Design review of the part shown in the three views and the two pictorial views. Dimensions are in mm from the part's minimum x, y and z. A direction names the side the tool comes from. Round coordinates to 2 decimals unless told otherwise and drop trailing zeros. Loops run counter-clockwise (first coordinate to the right, second up) from the corner with the lowest first, then second, coordinate; pieces in that order, holes last. Notation, with made-up numbers: M 57.25,59 L 96.25,59 A33 ccw 96.25,95 Z; hole C 1.25,-24.75 d7. An arc over 180 degrees is marked long. Answer in a Markdown table with one row per item. Add a question column.
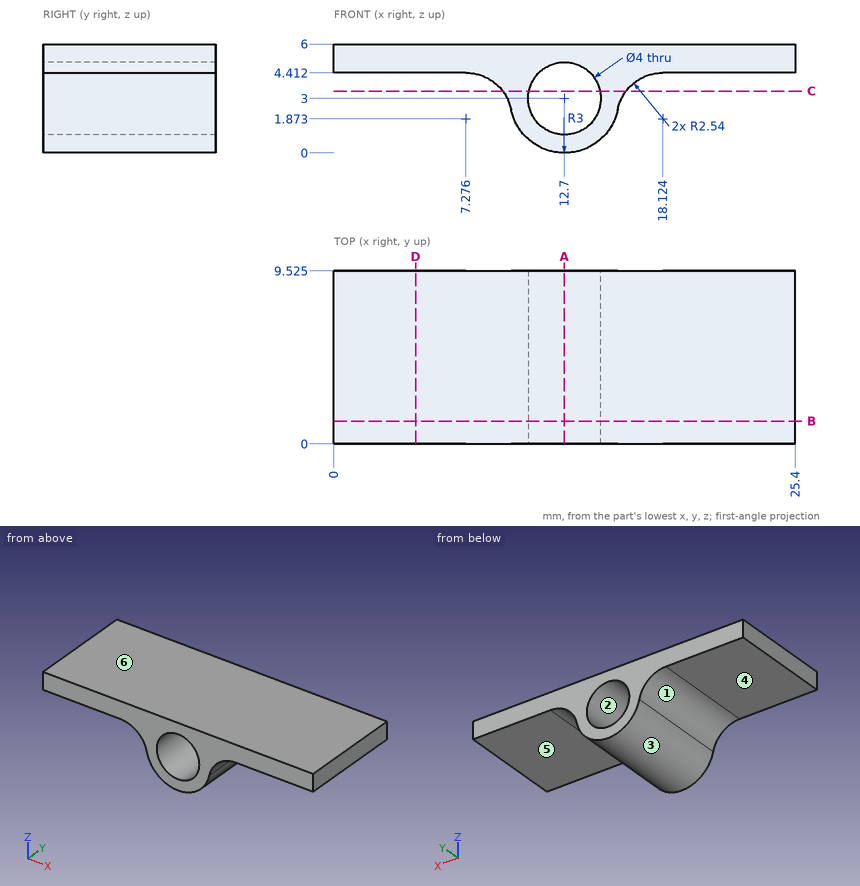
1. Take a section at B-B, the plane y = 1.25. State the section outline as (x, z) points (1 decimal).
2. Mouldability with a two-part tool opening along X and no side actions: class the marked faces 1, 2, 3 and 4 as released by +X, released by -X, zero draft, split by the parting line, or undercut.
3. For pin 1 Ø1.5 at (x, y) = (3, 8) entering from -Z; pin 2 Ø2 at (y, z) = (6, 2.5) entering from +X (1 decimal); pin 3 Ø1 at (x, z) = (9.5, 4) entering from -Y, all flat-tipped, find the tip position at first contact; note any pin that passes through.
4. Take a section at A-A, the plane x = 12.7. State the section outline as (y, z) points (1 decimal).
5. Machinability: for the marked faces 5 and 6, which of the approach directions +Z, -Z, +X, -X, +Y, -Y give a long, thin tool a straight path to every point of the face, cutting with its end or side? Answer none if there is none.
6. Take a section at D-D, the plane x = 4.5. State the section outline as (y, z) points (1 decimal), and give its area (3 significant figures).
7. Take a section at C-C, the plane z = 3.4. State the section outline as (x, y) points (1 decimal).
8. To check wall thickness, follow probe 1 along Z at (x, y) = (2.25, 3.75); probe 2 along X at (y, z) = (3.25, 3); probe 3 along X at (y, z) = (2.5, 2.5) (1 decimal). State the ranges of each line that lie inside material, in increasing order.
Check sheet entries:
| question | item | result |
|---|---|---|
| 1 | outline | M 0,4.4 L 7.3,4.4 A2.5 cw 9.8,2.4 A3 ccw 15.6,2.4 A2.5 cw 18.1,4.4 L 25.4,4.4 L 25.4,6 L 0,6 Z; hole C 12.7,3 d4 |
| 2 | face 1 | released by -X |
| 2 | face 2 | undercut |
| 2 | face 3 | split by the parting line |
| 2 | face 4 | zero draft |
| 3 | pin 1 | stops at z = 4.41 |
| 3 | pin 2 | stops at x = 16.2 |
| 3 | pin 3 | stops at y = 0 |
| 4 | outline | M 0,0 L 9.5,0 L 9.5,1 L 0,1 Z; M 0,5 L 9.5,5 L 9.5,6 L 0,6 Z |
| 5 | face 5 | -Z, +X, +Y, -Y |
| 5 | face 6 | +Z, +X, -X, +Y, -Y |
| 6 | outline | M 0,4.4 L 9.5,4.4 L 9.5,6 L 0,6 Z |
| 6 | area | 15.1 mm^2 |
| 7 | outline | M 9.3,0 L 10.7,0 L 10.7,9.5 L 9.3,9.5 Z; M 14.7,0 L 16.1,0 L 16.1,9.5 L 14.7,9.5 Z |
| 8 | probe 1 | z = 4.41 to 6 |
| 8 | probe 2 | x = 9.55 to 10.7, 14.7 to 15.85 |
| 8 | probe 3 | x = 9.7 to 10.8, 14.6 to 15.7 |
